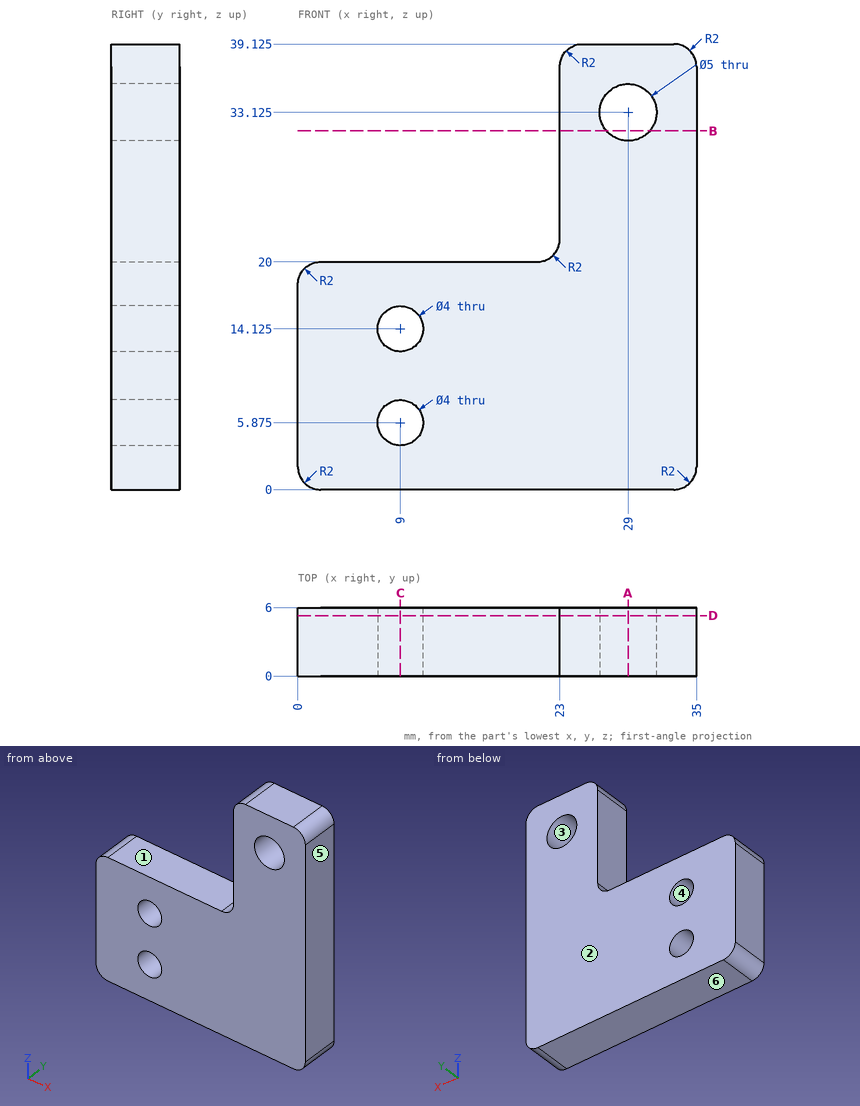
Study the drawing (mm; zero at the part's minimum x, y, z) and answer. A direction names the side the tool comes from. Give positions to 0.01 mm unless a question says otherwise; leave off trailing zeros. Write each loop counter-clockwise with the first axis right and the second up, starting at its lowest first coordinate (ties: lowest second). Pieces come first, ordered by that corner, then holes. Notation, with made-up numbers: (42, -20.5) - (101, -20.5) arc R21 ccw to (101, -16.5) - close; hole circle Ø4 at (1.5, 55.25). An arc over 180 degrees is marked (long way). Write item = value, one per line. Start each with the question number.
Item 1: Find section B-B (z = 31.5). Give the vertices of the cut face in (x, y).
Item 2: Find section D-D (y = 5.3). Give the vertices of the cut face in (x, z) (3 decimals).
Item 3: The mould has two halves that part along X. Classify the marked faces 3, 4, 5 and 6: +X half, -X half, draft (parallel to the pull), parting line (faces both ways), or undercut.
Item 4: A tool of negligible diameter and unlimited length cuts with its end or side. For the marked faces 1 and 2, from which of +Z, -Z, +X, -X, +Y, -Y can it reach the whole face along a straight path? Write none if from no direction.
Item 5: Each of these flat-tipped pins is pushed along its axis until it touches: P1, Ø1, axis at y = 4.5, z = 33, coming from the -X side; P2, Ø5, axis at x = 9, z = 14.125, coming from the -Y side; P3, Ø1.5, axis at y = 3, z = 20.5, coming from the -X side; P4, Ø2, axis at x = 12.5, y = 1, coming from the +Z side. Where does it stop, or does it pass through?
Item 6: Find section A-A (x = 29). Give the vertices of the cut face in (y, z) (3 decimals), then the cut area to 3 significant figures.
Item 7: Find the intervals of material crossed by probe 1 along Z at (x, y) = (9, 3.35) (3 decimals); probe 2 along X at (y, z) = (5.25, 33); probe 3 along Z at (x, y) = (29, 1.5) (3 decimals), in increasing order. Write a range as [from, to].
Item 8: Find section C-C (x = 9). Give the vertices of the cut face in (y, z) (3 decimals).
Response:
q1.outline = (23, 0) - (27.1, 0) - (27.1, 6) - (23, 6) - close; (30.9, 0) - (35, 0) - (35, 6) - (30.9, 6) - close
q2.outline = (0, 2) arc R2 ccw to (2, 0) - (33, 0) arc R2 ccw to (35, 2) - (35, 37.125) arc R2 ccw to (33, 39.125) - (25, 39.125) arc R2 ccw to (23, 37.125) - (23, 22) arc R2 cw to (21, 20) - (2, 20) arc R2 ccw to (0, 18) - close; hole circle Ø4 at (9, 5.875); hole circle Ø4 at (9, 14.125); hole circle Ø5 at (29, 33.125)
q3.face_3 = undercut
q3.face_4 = undercut
q3.face_5 = +X half
q3.face_6 = draft
q4.face_1 = +Z, -X, +Y, -Y
q4.face_2 = +Z, -Z, +X, -X, +Y
q5.P1 = 23
q5.P2 = 0
q5.P3 = 1.03
q5.P4 = 20
q6.outline = (0, 0) - (6, 0) - (6, 30.625) - (0, 30.625) - close; (0, 35.625) - (6, 35.625) - (6, 39.125) - (0, 39.125) - close
q6.area = 205 mm²
q7.probe_1 = [0, 3.875], [7.875, 12.125], [16.125, 20]
q7.probe_2 = [23, 26.5], [31.5, 35]
q7.probe_3 = [0, 30.625], [35.625, 39.125]
q8.outline = (0, 0) - (6, 0) - (6, 3.875) - (0, 3.875) - close; (0, 7.875) - (6, 7.875) - (6, 12.125) - (0, 12.125) - close; (0, 16.125) - (6, 16.125) - (6, 20) - (0, 20) - close
